Autodesk Inventor part; units mm, degrees
ref_plane "YZ Plane" through (0, 0, 0) normal (1, 0, 0) x (0, 1, 0)
ref_plane "XZ Plane" through (0, 0, 0) normal (0, 1, 0) x (-1, 0, 0)
ref_plane "XY Plane" through (0, 0, 0) normal (0, 0, 1) x (1, 0, 0)
sketch "Sketch1" plane through (0, 0, 0) normal (0, 0, 1) x (1, 0, 0)
  circle A0 centre (0, 0) radius 34
  dimension "d0" = 68
extrude "Extrusion1" add sketch "Sketch1" against normal blind 2.54
sketch "Sketch3" plane through (0, 0, -2.54) normal (0, 0, -1) x (-1, 0, 0)
  circle A0 centre (0, 0) radius 26 construction
  line L0 (3, -24) -> (-3, -24)
  line L1 (-3, -24) -> (-3, -28)
  line L2 (-3, -28) -> (3, -28)
  line L3 (3, -28) -> (3, -24)
  line L4 (3, -24) -> (-3, -28) construction
  line L5 (-3, -24) -> (3, -28) construction
  line L6 (8.648, -26.7995) -> (14.1293, -24.3591)
  line L7 (14.1293, -24.3591) -> (12.5023, -20.7049)
  line L8 (7.021, -23.1453) -> (8.648, -26.7995)
  line L9 (12.5023, -20.7049) -> (7.021, -23.1453)
  line L10 (18.8007, -20.9651) -> (22.8154, -16.5062)
  line L11 (22.8154, -16.5062) -> (19.8429, -13.8297)
  line L12 (15.8281, -18.2886) -> (18.8007, -20.9651)
  line L13 (19.8429, -13.8297) -> (15.8281, -18.2886)
  line L14 (25.7025, -11.5056) -> (27.5566, -5.7993)
  line L15 (27.5566, -5.7993) -> (23.7524, -4.5632)
  line L16 (21.8983, -10.2696) -> (25.7025, -11.5056)
  line L17 (23.7524, -4.5632) -> (21.8983, -10.2696)
  line L18 (28.1602, -0.0568) -> (27.533, 5.9104)
  line L19 (27.533, 5.9104) -> (23.5549, 5.4922)
  line L20 (24.1821, -0.4749) -> (28.1602, -0.0568)
  line L21 (23.5549, 5.4922) -> (24.1821, -0.4749)
  line L22 (25.7487, 11.4019) -> (22.7487, 16.5981)
  line L23 (22.7487, 16.5981) -> (19.2846, 14.5981)
  line L24 (22.2846, 9.4019) -> (25.7487, 11.4019)
  line L25 (19.2846, 14.5981) -> (22.2846, 9.4019)
  line L26 (18.885, 20.8891) -> (14.0309, 24.4158)
  line L27 (14.0309, 24.4158) -> (11.6798, 21.1798)
  line L28 (16.5339, 17.6531) -> (18.885, 20.8891)
  line L29 (11.6798, 21.1798) -> (16.5339, 17.6531)
  line L30 (8.756, 26.7644) -> (2.8871, 28.0119)
  line L31 (2.8871, 28.0119) -> (2.0554, 24.0993)
  line L32 (7.9243, 22.8518) -> (8.756, 26.7644)
  line L33 (2.0554, 24.0993) -> (7.9243, 22.8518)
  line L34 (-2.8871, 28.0119) -> (-8.756, 26.7644)
  line L35 (-8.756, 26.7644) -> (-7.9243, 22.8518)
  line L36 (-2.0554, 24.0993) -> (-2.8871, 28.0119)
  line L37 (-7.9243, 22.8518) -> (-2.0554, 24.0993)
  line L38 (-14.0309, 24.4158) -> (-18.885, 20.8891)
  line L39 (-18.885, 20.8891) -> (-16.5339, 17.6531)
  line L40 (-11.6798, 21.1798) -> (-14.0309, 24.4158)
  line L41 (-16.5339, 17.6531) -> (-11.6798, 21.1798)
  line L42 (-22.7487, 16.5981) -> (-25.7487, 11.4019)
  line L43 (-25.7487, 11.4019) -> (-22.2846, 9.4019)
  line L44 (-19.2846, 14.5981) -> (-22.7487, 16.5981)
  line L45 (-22.2846, 9.4019) -> (-19.2846, 14.5981)
  line L46 (-27.533, 5.9104) -> (-28.1602, -0.0568)
  line L47 (-28.1602, -0.0568) -> (-24.1821, -0.4749)
  line L48 (-23.5549, 5.4922) -> (-27.533, 5.9104)
  line L49 (-24.1821, -0.4749) -> (-23.5549, 5.4922)
  line L50 (-27.5566, -5.7993) -> (-25.7025, -11.5056)
  line L51 (-25.7025, -11.5056) -> (-21.8983, -10.2696)
  line L52 (-23.7524, -4.5632) -> (-27.5566, -5.7993)
  line L53 (-21.8983, -10.2696) -> (-23.7524, -4.5632)
  line L54 (-22.8154, -16.5062) -> (-18.8007, -20.9651)
  line L55 (-18.8007, -20.9651) -> (-15.8281, -18.2886)
  line L56 (-19.8429, -13.8297) -> (-22.8154, -16.5062)
  line L57 (-15.8281, -18.2886) -> (-19.8429, -13.8297)
  line L58 (-14.1293, -24.3591) -> (-8.648, -26.7995)
  line L59 (-8.648, -26.7995) -> (-7.021, -23.1453)
  line L60 (-12.5023, -20.7049) -> (-14.1293, -24.3591)
  line L61 (-7.021, -23.1453) -> (-12.5023, -20.7049)
  point P0 (0, -26)
  dimension "d6" = 52
  dimension "d7" = 4
  dimension "d8" = 6
  dimension "d11" = 360
extrude "Extrusion3" cut sketch "Sketch3" against normal through all
sketch "Sketch7" plane through (0, 0, 0) normal (0, 0, 1) x (1, 0, 0)
  line L0 (-48.5775, -37.85) -> (48.5775, -37.85)
  line L1 (48.5775, -37.85) -> (48.5775, 37.85)
  line L2 (48.5775, 37.85) -> (-48.5775, 37.85)
  line L3 (-48.5775, 37.85) -> (-48.5775, -37.85)
  line L4 (-48.5775, -37.85) -> (48.5775, 37.85) construction
  line L5 (48.5775, -37.85) -> (-48.5775, 37.85) construction
  circle A0 centre (0, 0) radius 34
  dimension "mountWidth" = 97.155
  dimension "mountHeight" = 75.7
extrude "Extrusion4" add sketch "Sketch7" against normal blind 2.54
sketch "Sketch8" plane through (0, 0, 0) normal (0, 0, 1) x (1, 0, 0)
  line L0 (-42.2275, -31.5) -> (42.2275, -31.5) construction
  line L1 (42.2275, -31.5) -> (42.2275, 31.5) construction
  line L2 (42.2275, 31.5) -> (-42.2275, 31.5) construction
  line L3 (-42.2275, 31.5) -> (-42.2275, -31.5) construction
  line L4 (-48.5775, -37.85) -> (48.5775, -37.85) construction
  line L5 (-48.5775, 37.85) -> (-48.5775, -37.85) construction
  line L6 (48.5775, -37.85) -> (48.5775, 37.85) construction
  line L7 (48.5775, 37.85) -> (-48.5775, 37.85) construction
  point P0 (0, 0)
  dimension "d47" = 6.35
  dimension "d48" = 6.35
  dimension "d49" = 6.35
  dimension "d50" = 6.35
sketch "Sketch10" plane through (0, 0, 0) normal (0, 0, 1) x (1, 0, 0)
  circle A0 centre (0, 0) radius 12.7
  dimension "d58" = 25.4
extrude "Extrusion5" cut sketch "Sketch10" against normal through all
sketch "Sketch11" plane through (0, 0, 0) normal (0, 0, 1) x (1, 0, 0)
  circle A0 centre (-42.2275, 31.5) radius 2.5527
  circle A1 centre (-42.2275, 31.5) radius 3.175
  circle A2 centre (42.2275, 31.5) radius 2.5527
  circle A3 centre (42.2275, 31.5) radius 3.175
  circle A4 centre (42.2275, -31.5) radius 2.5527
  circle A5 centre (42.2275, -31.5) radius 3.175
  circle A6 centre (-42.2275, -31.5) radius 2.5527
  circle A7 centre (-42.2275, -31.5) radius 3.175
  point P0 (0, 0)
  dimension "d61" = 6.35
extrude "Extrusion6" cut sketch "Sketch11" against normal through all contours A0 | A1 | A2 | A3 | A4 | A5 | A6 | A7
equation "\"d1\" = CoverDepth"
equation "\"d6\" = 2 * LightRingCenterRadius"
equation "\"depth\" = CoverDepth"
properties part number "2020LightRingCover" material "Polycarbonate, Clear"
The listing builds one solid part. Answer for the finished solid, in the listing's coordinates (mm). Give positions to 0.01 mm unless a question says otherwise; leave off trailing zeros. Order: outer loops, then holes, each group sorted by start corner. A loop starts at its lowest first (then second) coordinate and runs counter-clockwise, first axis right, second up. Notation, with made-up numbers: (-31.5, 46) -> (-8.5, 46) arc R17 ccw to (-8.5, 79) -> close; hole circle Ø5 at (52, -8.75). An arc over 180 degrees is marked (long way). Answer as a JSON object with one key per item and string values. Group by question number.
Item 1: Consider L1, parallel to Y at x = 0, z = -1.55; L2, parallel to Y at x = -25, z = -0.6; L3, parallel to X at y = -18, z = -1.15. Determine where each line is inside the solid, lowest interval first. Write a range as from..to.
Item 2: The part is cut by section A-A on y = 31.5. Write down the section's boundary in (x, z).
Item 3: The part is cut by section B-B on x = 0. Write down the section's boundary in (y, z).
Item 4: Flat-ended cylindrical pins translate along their axes: pin 1 (8 mm diameter, centred on x = -22, y = -17, fed in from -Z); pin 2 (5 mm diameter, centred on x = 42.23, y = 31.5, fed in from -Z). Find the tip coordinate at first contact, or state that the pin passes through.
Item 5: Determine the mould class of faces 1 (the flat face through (-14.073, 19.441, -1.288)), 2 (the flat face through (48.578, -1, -1)) for opening direction Y: pulls with the +Y half, pulls with the -Y half, needs draft (parallel to the pull), parting line crosses it, or undercut.
Item 6: The part is cut by section C-C on z = -1.1. Give the number of separate pieces and of enclosed holes in the cut face, and give its area (3 significant figures).
Result set:
{
 "1": {"L1": "-37.85..-28, -24..-12.7, 12.7..37.85", "L2": "-37.85..-11.28, -4.97..-0.39, 5.64..10.97, 12.7..37.85", "L3": "-48.58..-21.47, -16.09..16.09, 21.47..48.58"},
 "2": {"outline": "(-48.58, -2.54) -> (-45.4, -2.54) -> (-45.4, 0) -> (-48.58, 0) -> close; (-39.05, -2.54) -> (39.05, -2.54) -> (39.05, 0) -> (-39.05, 0) -> close; (45.4, -2.54) -> (48.58, -2.54) -> (48.58, 0) -> (45.4, 0) -> close"},
 "3": {"outline": "(-37.85, -2.54) -> (-28, -2.54) -> (-28, 0) -> (-37.85, 0) -> close; (-24, -2.54) -> (-12.7, -2.54) -> (-12.7, 0) -> (-24, 0) -> close; (12.7, -2.54) -> (37.85, -2.54) -> (37.85, 0) -> (12.7, 0) -> close"},
 "4": {"pin 1": "z = -2.54", "pin 2": "through"},
 "5": {"face 1": "undercut", "face 2": "needs draft"},
 "6": {"separate pieces": "1", "enclosed holes": "20", "area": "6,360 mm²"}
}
